```python
from build123d import *

# Parameters (mm, degrees)
SKETCH1_R                      = 14.6812
SKETCH1_R_2                    = 11.5062
BEARING_INSERT_EXTRUDE_DEPTH   = 4.7625
APEX_SLOT_INSERT_EXTRUDE_DEPTH = 3.175
FILLET1_R                      = 16.002
FILLET2_R                      = 2.54


with BuildPart() as part:
    # Sketch1 → Bearing_Insert_Extrude (new, symmetric)
    with BuildSketch(Plane(origin=(0, 0, 0), x_dir=(1, 0, 0), z_dir=(0, 1, 0))):
        with Locations(Location((0, 0, 0), (0, 0, 90))):
            Circle(SKETCH1_R)
        with Locations(Location((0, 0, 0), (0, 0, 90))):
            Circle(SKETCH1_R_2, mode=Mode.SUBTRACT)
    extrude(amount=BEARING_INSERT_EXTRUDE_DEPTH, both=True)

    # Sketch1<4> → Apex_Slot_Insert_Extrude (add, symmetric)
    # profile 1 of 2: a face of its own
    with BuildSketch(Plane(origin=(0, 0, 0), x_dir=(1, 0, 0), z_dir=(0, 1, 0))):
        with BuildLine():
            Line((-10.31875, -10.443228997), (-10.31875, -49.3903))
            Line((-10.31875, -49.3903), (10.31875, -49.3903))
            Line((10.31875, -49.3903), (10.31875, -37.376828003))
            Line((10.31875, -37.376828003), (16.482194895, -47.68873648))
            Line((16.482194895, -47.68873648), (34.196641747, -37.100782052))
            Line((34.196641747, -37.100782052), (14.215063896, -3.670094259))
            ThreePointArc((14.215063896, -3.670094259), (3.906936657, -14.151801278), (-10.31875, -10.443228997))
        make_face()
        with BuildLine():
            ThreePointArc((5.55625, -39.07155), (0, -44.6278), (-5.55625, -39.07155))
            Line((-5.55625, -39.07155), (-5.55625, -25.48255))
            ThreePointArc((-5.55625, -25.48255), (0, -19.9263), (5.55625, -25.48255))
            Line((5.55625, -25.48255), (5.55625, -39.07155))
        make_face(mode=Mode.SUBTRACT)
        with BuildLine():
            ThreePointArc((24.81471526, -30.686932725), (22.896044222, -38.306809993), (15.276166955, -36.388138955))
            Line((15.276166955, -36.388138955), (8.304406193, -24.723857028))
            ThreePointArc((8.304406193, -24.723857028), (10.22307723, -17.10397976), (17.842954497, -19.022650798))
            Line((17.842954497, -19.022650798), (24.81471526, -30.686932725))
        make_face(mode=Mode.SUBTRACT)
    # profile 2 of 2: a face of its own
    with BuildSketch(Plane(origin=(0, 0, 0), x_dir=(1, 0, 0), z_dir=(0, 1, 0))):
        Polygon((10.31875, -49.3903), (10.31875, -37.376828003), (16.482194895, -47.68873648), align=None)
    extrude(amount=APEX_SLOT_INSERT_EXTRUDE_DEPTH, both=True)

    # Fillet1
    fillet1_edges = [part.edges().sort_by_distance(p)[0] for p in [
        (14.215063896, 0, 3.670094259),
        (-10.31875, 0, 10.443228997),
    ]]
    fillet(fillet1_edges, radius=FILLET1_R)

    # Fillet2
    fillet2_edges = [part.edges().sort_by_distance(p)[0] for p in [
        (-10.31875, 0, 49.3903),
        (10.31875, 0, 49.3903),
        (16.482194895, 0, 47.68873648),
        (34.196641747, 0, 37.100782052),
    ]]
    fillet(fillet2_edges, radius=FILLET2_R)


solid = part.part
```
For this review, take the finished solid that the model builds, in its own axes (mm). A direction names the side the tool comes from. Give positions to 0.01 mm unless a question says otherwise; leave off trailing zeros. Order: outer loops, then holes, each group sorted by start corner. A loop starts at its lowest first (then second) coordinate and runs counter-clockwise, first axis right, second up.
1) The part is to be moulded in two halves that separate along Z. For faces 4 (the face through (33.17, 0.04, 36.87)), 5 (the face through (1, 0, 49.39)), 6 (the face through (0.122, 0.044, 44.626)), say which applies: released by +Z, released by -Z, zero draft, split by the parting line, or undercut.
2) Take a section at D-D (z = 21.5). Give the boundary of the cut face in (x, y) (3 decimals).
3) Take a section at B-B (y = -2). Give the boundary of the cut face in (x, z), then the cut area to 3 significant figures.
4) Take a section at C-C (z = -3). Give the boundary of the cut face in (x, y).
5) Wall thickness on line 1 (Z direction, x = -4, y = -2); line 2 (X direction, y = -2.5, z = 0); line 3 (X direction, y = -0.25, z = 4): over which ranges is each line inside the solid? List them lowest first.
6) Take a section at A-A (x = 0). Give the boundary of the cut face in (y, z) (1 decimal).
7) Insertion check: pin 1 (3 mm diameter, centred on y = -1.5, z = 30, fed in from -X); pin 2 (20.5 mm diameter, centred on x = 0, z = 0, fed in from +Y); pin 3 (2 mm diameter, centred on x = 14.5, y = 0, fed in from +Z); pin 4 (12 mm diameter, centred on x = 4.5, z = 33, fed in from -Y) (3 decimals). Each pin has a flat end and moves straight along its axis. Give the tip position at first contact, or say it passes through.
8) For faces 1 (the face through (21.28, 0.04, 24.77)), 2 (the face through (8, 4.762, 9)), 3 (the face through (-10.319, 0, 31)), list the 3-axis set-ups (+Z, -Z, +X, -X, +Y, -Y) from which the entire face can be reached by the end or side of a thin tool; tool diameter is ignored.
Derived:
1. face 4: split by the parting line
1. face 5: released by +Z
1. face 6: undercut
2. outline: (-10.319, -3.175) - (-3.874, -3.175) - (-3.874, 3.175) - (-10.319, 3.175) - close; (3.874, -3.175) - (7.53, -3.175) - (7.53, 3.175) - (3.874, 3.175) - close; (19.324, -3.175) - (24.872, -3.175) - (24.872, 3.175) - (19.324, 3.175) - close
3. outline: (-12.59, 7.55) arc R14.68 ccw (long way) to (14.68, 0.02) arc R16 cw to (16.95, 8.24) - (32.89, 34.92) arc R2.54 ccw to (32.02, 38.4) - (16.78, 47.51) arc R2.54 ccw to (16.15, 47.78) - (10.65, 49.3) arc R2.54 ccw to (9.97, 49.39) - (-7.78, 49.39) arc R2.54 ccw to (-10.32, 46.85) - (-10.32, 15.77) arc R16 cw to start; hole circle Ø23.01 at (0, 0); hole (-5.56, 25.48) arc R5.56 ccw to (5.56, 25.48) - (5.56, 39.07) arc R5.56 ccw to (-5.56, 39.07) - close; hole (8.3, 24.72) arc R5.56 ccw to (17.84, 19.02) - (24.81, 30.69) arc R5.56 ccw to (15.28, 36.39) - close
3. area: 1,120 mm2
4. outline: (-14.37, -4.76) - (-11.11, -4.76) - (-11.11, 4.76) - (-14.37, 4.76) - close; (11.11, -4.76) - (14.37, -4.76) - (14.37, 4.76) - (11.11, 4.76) - close
5. line 1: z = -14.13 to -10.79, 10.79 to 21.63, 42.93 to 49.39
5. line 2: x = -14.68 to -11.51, 11.51 to 14.68
5. line 3: x = -14.13 to -10.79, 10.79 to 15.18
6. outline: (-4.8, -14.7) - (4.8, -14.7) - (4.8, -11.5) - (-4.8, -11.5) - close; (-4.8, 11.5) - (4.8, 11.5) - (4.8, 14.7) - (3.2, 14.7) - (3.2, 19.9) - (-3.2, 19.9) - (-3.2, 14.7) - (-4.8, 14.7) - close; (-3.2, 44.6) - (3.2, 44.6) - (3.2, 49.4) - (-3.2, 49.4) - close
7. pin 1: stops at x = -10.32
7. pin 2: passes through
7. pin 3: stops at z = 48.51
7. pin 4: stops at y = -3.175
8. face 1: +Y, -Y
8. face 2: +Z, -Z, +X, -X, +Y
8. face 3: +Z, -X, +Y, -Y
